from build123d import *

# Parameters (mm, degrees)
F0_R      = 47.5
F1_DEPTH  = 4.5
F2_R      = 3.5
F3_DEPTH  = 114
F3_TAPER  = 0.2
F4_R      = 0.5
F5_R      = 38.002083118
F5_R_2    = 37.802083118
F6_DEPTH  = 0.2
F7_R      = 28.9679765701
F7_R_2    = 28.767975761
F8_DEPTH  = 0.2
F9_R      = 19.4251779467
F9_R_2    = 19.2251771527
F10_DEPTH = 0.2
F11_R     = 12.0890308172
F11_R_2   = 11.8890312486
F12_DEPTH = 0.2
F14_ANGLE = -90


with BuildPart() as f1:
    # F0 (on Front) → F1 (new body, symmetric)
    with BuildSketch(Plane.XZ):
        with Locations((0, 1.5224246528)):
            Circle(F0_R)
    extrude(amount=F1_DEPTH, both=True)

    # F2 (on Top) → F3 (join)
    with BuildSketch(Plane.XY):
        Circle(F2_R)
    extrude(amount=-F3_DEPTH, taper=F3_TAPER)

    # F4
    f4_edges = [f1.edges().sort_by_distance(p)[0] for p in [
        (-47.5, -4.5, 1.522425),
        (-47.5, 4.5, 1.522425),
    ]]
    fillet(f4_edges, radius=F4_R)

    # F5 (on face) → F6 (cut)
    with BuildSketch(Plane.XZ.offset(4.5)):
        with Locations((0, 1.5224246528)):
            Circle(F5_R)
        with Locations((0, 1.5224246528)):
            Circle(F5_R_2, mode=Mode.SUBTRACT)
    extrude(amount=-F6_DEPTH, mode=Mode.SUBTRACT)

    # F7 (on face) → F8 (cut)
    with BuildSketch(Plane.XZ.offset(4.5)):
        with Locations((0, 1.5499041183)):
            Circle(F7_R)
        with Locations((0, 1.5499041183)):
            Circle(F7_R_2, mode=Mode.SUBTRACT)
    extrude(amount=-F8_DEPTH, mode=Mode.SUBTRACT)

    # F9 (on face) → F10 (cut)
    with BuildSketch(Plane.XZ.offset(4.5)):
        with Locations((0, 1.613457338)):
            Circle(F9_R)
        with Locations((0, 1.613457338)):
            Circle(F9_R_2, mode=Mode.SUBTRACT)
    extrude(amount=-F10_DEPTH, mode=Mode.SUBTRACT)

    # F11 (on face) → F12 (cut)
    with BuildSketch(Plane.XZ.offset(4.5)):
        with Locations((0, 1.6672129277)):
            Circle(F11_R)
        with Locations((0, 1.6672129277)):
            Circle(F11_R_2, mode=Mode.SUBTRACT)
    extrude(amount=-F12_DEPTH, mode=Mode.SUBTRACT)


with BuildPart() as f1_1:
    # F14: moved
    add(f1.part.rotate(Axis((14.7541314363, 0, 0), (1, 0, 0)), F14_ANGLE))


solid = f1_1.part
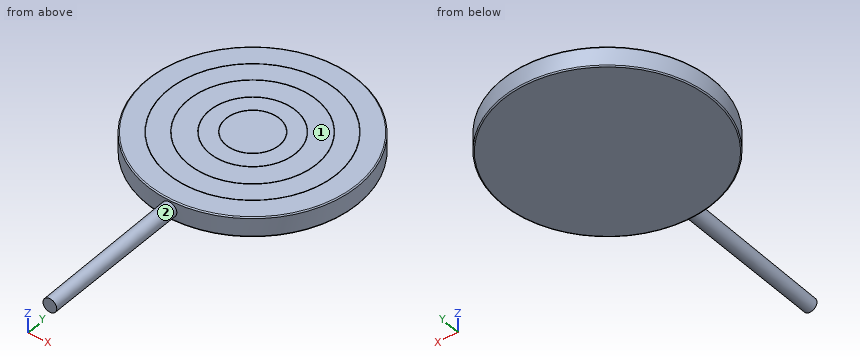
Here's how the part is built. I have some questions about the finished solid (model axes, mm). Face numbers are marked on the shaded views. A direction names the side the tool comes from. Round coordinates to 2 decimals unless told otherwise and drop trailing zeros. Loops run counter-clockwise (first coordinate to the right, second up) from the corner with the lowest first, then second, coordinate; pieces in that order, holes last. Notation, with made-up numbers: (-32.5, 1.5) - (22.5, 1.5) arc R18 cw to (22.5, 26.5) - close; hole circle Ø4 at (0.5, 26.5). An arc over 180 degrees is marked (long way). One line per question, with ' | ' between items. Start each with the question number.
Q1. Will these pins go through, and if not, where does the flat tip stop? pin 1 (4 mm diameter, centred on y = -75, z = -2.5, fed in from -X); pin 2 (1.5 mm diameter, centred on y = -81.5, z = -2.5, fed in from -X); pin 3 (1 mm diameter, centred on x = -24, z = 0.5, fed in from +Y).
Q2. For the marked faces 1 and 2, which set-ups out of +Z, -Z, +X, -X, +Y, -Y let a thin tool reach every point of the face, with its end or its side?
Q3. Please list where these lines run through material, in increasing order: line 1 (X direction, y = -100, z = 0.5); line 2 (X direction, y = -17.5, z = -3.5); line 3 (Y direction, x = 20, z = -1.5). Write a range as [from, to].
Q4. I want a section at A-A (y = -99.5). Write out the boundary of the cut face in (x, z).
Response values:
1) pin 1: stops at x = -3.2 | pin 2: stops at x = -2.7 | pin 3: stops at y = 42.8
2) face 1: +Z, +X, -X, +Y, -Y | face 2: -Y
3) line 1: x = [-3.11, 3.11] | line 2: x = [-43.52, 43.52] | line 3: y = [-41.56, 44.61]
4) outline: circle Ø6.31 at (0, 0)
